from build123d import *

# Parameters (mm, degrees)
F0_W      = 100
F0_H      = 45
F1_DEPTH  = 80
F3_DEPTH  = 20
F5_DEPTH  = 30
F6_W      = 20
F6_H      = 15
F7_DEPTH  = 20
F9_DEPTH  = 25.001
F11_DEPTH = 80.001


with BuildPart() as f1:
    # F0 (on Front) → F1 (new body)
    with BuildSketch(Plane.XZ):
        with Locations((50, 22.5)):
            Rectangle(F0_W, F0_H)
    extrude(amount=F1_DEPTH)

    # F2 (on face) → F3 (cut)
    with BuildSketch(Plane.XY.offset(45)):
        with BuildLine():
            Line((0, -80), (70, -80))
            ThreePointArc((70, -80), (49.4974746831, -30.5025253169), (0, -10))
            Line((0, -10), (0, -80))
        make_face()
    extrude(amount=-F3_DEPTH, mode=Mode.SUBTRACT)

    # F4 (on face) → F5 (cut)
    with BuildSketch(Plane.XY.offset(45)):
        with BuildLine():
            ThreePointArc((67.5, -15), (65.3033008589, -9.6966991411), (60, -7.5))
            ThreePointArc((60, -7.5), (54.6966991411, -20.3033008589), (67.5, -15))
        make_face()
    extrude(amount=-F5_DEPTH, mode=Mode.SUBTRACT)

    # F6 (on face) → F7 (join)
    with BuildSketch(Plane.XY.offset(25)):
        with Locations((10, -72.5)):
            Rectangle(F6_W, F6_H)
    extrude(amount=F7_DEPTH)

    # F8 (on face) → F9 (cut, through all)
    with BuildSketch(Plane.XY.offset(25)):
        with BuildLine():
            Line((35, -19.3782217351), (35, -50))
            Line((35, -50), (63.2455532034, -50))
            ThreePointArc((63.2455532034, -50), (51.4535762322, -32.5391793906), (35, -19.3782217351))
        make_face()
    extrude(amount=-F9_DEPTH, mode=Mode.SUBTRACT)

    # F10 (on face) → F11 (cut, through all)
    with BuildSketch(Plane.XZ.offset(80)):
        with BuildLine():
            ThreePointArc((83.6190264738, 45), (95.7773967757, 23.944395449), (100, 0))
            Line((100, 0), (100, 45))
            Line((100, 45), (83.6190264738, 45))
        make_face()
    extrude(amount=-F11_DEPTH, mode=Mode.SUBTRACT)


solid = f1.part
Build history of the part. All positions in model axes, mm. A direction names the side the tool comes from. Coordinates: 2 decimals unless noted, no trailing zeros. Order: outer loops, then holes, each group sorted by start corner. A loop starts at its lowest first (then second) coordinate and runs counter-clockwise, first axis right, second up. Notation, with made-up numbers: M -31.5,56 L 1.5,56 A13 cw 1.5,75 Z; hole C 78.5,36 d6. An arc over 180 degrees is marked long. One line per question, with ' | ' between items. Start each with the question number.
Q1. Saw through at C-C (y = -45.5). List the corners of the cut face in (x, z).
Q2. Saw through at D-D (x = 60). List the corners of the cut face in (y, z), then the cut area to 3 significant figures.
Q3. Flat gauge pins, fed straight in: pin 1 Ø6 at (x, y) = (48.5, -48.5) entering from +Z; pin 2 Ø16.5 at (y, z) = (-75.5, 36.5) entering from +X; pin 3 Ø4.5 at (x, y) = (61, -13.5) entering from +Z. Where does each tip first touch, or does it go through?
Q4. Saw through at A-A (z = 29). List the corners of the cut face in (x, y), then the cut area to 3 significant figures.
Q5. Saw through at B-B (x = 38.5). List the corners of the cut face in (y, z), then the cut area to 3 significant figures.
Q6. Probe L1, parallel to Y at x = 60, z = 38.75; L2, parallel to X at y = -15, z = 28.75; L3, parallel to Z at x = 58, y = -60. List the from-to ranges inside material, lowest first. Write a range as from..to.
Q7. Two-plate mould, pull along Y, no slides. Class faces 1 (the face through (52.564, -15.976, 30.21)), 2 (the face through (27, -45, 25)), 3 (the face through (20, -73, 35)), 4 (the face through (49, -80, 17)): +Y half, -Y half, draft (parallel to the pull), parting line (faces both ways), or undercut.
Q8. 3-axis set-ups, long thin cutter, end or side, ignore diameter. For faces 5 (the face through (60, -31, 45)), 6 (the face through (60, -15, 15)), 7 (the face through (35, -34, 13)), 8 (the face through (10, -65, 35)): which of +Z, -Z, +X, -X, +Y, -Y reach the whole face in a straight line?
Check values:
1) outline: M 0,0 L 35,0 L 35,25 L 0,25 Z; M 60.91,0 L 100,0 A70 ccw 83.62,45 L 60.91,45 Z
2) outline: M -80,0 L -50,0 L -50,25 L -80,25 Z; M -43.94,0 L 0,0 L 0,45 L -7.5,45 L -7.5,15 L -22.5,15 L -22.5,45 L -43.94,45 Z | area: 2,280 mm2
3) pin 1: stops at z = 25 | pin 2: stops at x = 94.05 | pin 3: stops at z = 15
4) outline: M 0,-80 L 20,-80 L 20,-65 L 0,-65 Z; M 0,-10 A70 cw 70,-80 L 93.71,-80 L 93.71,0 L 0,0 Z; hole C 60,-15 d15 | area: 3,770 mm2
5) outline: M -80,0 L -50,0 L -50,25 L -80,25 Z; M -21.54,0 L 0,0 L 0,45 L -21.54,45 Z | area: 1,720 mm2
6) L1: y = -43.94..-22.5, -7.5..0 | L2: x = 25.98..52.5, 67.5..93.82 | L3: z = 0..25
7) face 1: undercut | face 2: undercut | face 3: draft | face 4: -Y half
8) face 5: +Z, +X, -X, +Y, -Y | face 6: +Z | face 7: +Z, -Z | face 8: +Z, -X
